from build123d import *

# Parameters (mm, degrees)
F0_W     = 125
F0_H     = 75
F1_DEPTH = 5
F2_DEPTH = 2.5
F3_R     = 2.405164
F3_R_2   = 2.5
F4_DEPTH = 5


with BuildPart() as f1:
    # F0 (on Top) → F1 (new body, symmetric)
    with BuildSketch(Plane.XY):
        Rectangle(F0_W, F0_H)
        Polygon((-55, 26), (-55, 30), (-53, 30), (-48, 30), (-46, 30), (-41, 30), (-39, 30), (-34, 30), (-32, 30), (-27, 30), (-25, 30), (-20, 30), (-18, 30), (-13, 30), (-11, 30), (-6, 30), (-4, 30), (1, 30), (3, 30), (8, 30), (10, 30), (15, 30), (17, 30), (22, 30), (24, 30), (29, 30), (31, 30), (36, 30), (38, 30), (43, 30), (45, 30), (55, 30), (55, 20.999727), (55, 18.999727), (55, 13.999727), (55, 11.999727), (55, 6.999727), (55, 4.999727), (55, -0.000273), (55, -2.000273), (55, -7.000273), (55, -9.000273), (55, -14.000273), (55, -16.000273), (55, -21.000273), (55, -23.000273), (55, -28), (55, -30), (50, -30), (48, -30), (43, -30), (41, -30), (36, -30), (34, -30), (29, -30), (27, -30), (22, -30), (20, -30), (15, -30), (13, -30), (8, -30), (6, -30), (1, -30), (-1, -30), (-6, -30), (-8, -30), (-13, -30), (-15, -30), (-20, -30), (-22, -30), (-27, -30), (-29, -30), (-34, -30), (-36, -30), (-41, -30), (-43, -30), (-48, -30), (-50, -30), (-55, -30), (-55, -25), (-55, -23), (-55, -18), (-55, -16), (-55, -11), (-55, -9), (-55, -4), (-55, -2), (-55, 3), (-55, 5), (-55, 10), (-55, 12), (-55, 17), (-55, 19), (-55, 24), align=None, mode=Mode.SUBTRACT)
    extrude(amount=F1_DEPTH, both=True)

    # F0 (on Top) → F2 (join, symmetric)
    with BuildSketch(Plane.XY):
        Polygon((-48, -30), (-55, -23), (-55, -25), (-50, -30), align=None)
        Polygon((-41, -30), (-55, -16), (-55, -18), (-43, -30), align=None)
        Polygon((-34, -30), (-55, -9), (-55, -11), (-36, -30), align=None)
        Polygon((-27, -30), (-55, -2), (-55, -4), (-29, -30), align=None)
        Polygon((-20, -30), (-55, 5), (-55, 3), (-22, -30), align=None)
        Polygon((-13, -30), (-55, 12), (-55, 10), (-15, -30), align=None)
        Polygon((-6, -30), (-55, 19), (-55, 17), (-8, -30), align=None)
        Polygon((1, -30), (-55, 26), (-55, 24), (-1, -30), align=None)
        Polygon((-53, 30), (-55, 30), (6, -30), (8, -30), align=None)
        Polygon((-46, 30), (-48, 30), (13, -30), (15, -30), align=None)
        Polygon((-39, 30), (-41, 30), (20, -30), (22, -30), align=None)
        Polygon((-32, 30), (-34, 30), (27, -30), (29, -30), align=None)
        Polygon((-25, 30), (-27, 30), (34, -30), (36, -30), align=None)
        Polygon((-18, 30), (-20, 30), (41, -30), (43, -30), align=None)
        Polygon((-11, 30), (-13, 30), (48, -30), (50, -30), align=None)
        Polygon((3, 30), (1, 30), (55, -23.000273), (55, -21.000273), align=None)
        Polygon((10, 30), (8, 30), (55, -16.000273), (55, -14.000273), align=None)
        Polygon((45, 30), (43, 30), (55, 18.999727), (55, 20.999727), align=None)
        Polygon((38, 30), (36, 30), (55, 11.999727), (55, 13.999727), align=None)
        Polygon((31, 30), (29, 30), (55, 4.999727), (55, 6.999727), align=None)
        Polygon((24, 30), (22, 30), (55, -2.000273), (55, -0.000273), align=None)
        Polygon((17, 30), (15, 30), (55, -9.000273), (55, -7.000273), align=None)
        Polygon((-4, 30), (-6, 30), (55, -30), (55, -28), align=None)
    extrude(amount=F2_DEPTH, both=True)

    # F3 (on face) → F4 (join)
    with BuildSketch(Plane(origin=(0, 0, -5), x_dir=(1, 0, 0), z_dir=(0, 0, -1))):
        with Locations((-57.5, 32.5)):
            Circle(F3_R)
        with Locations((57.5, 32.5)):
            Circle(F3_R_2)
        with Locations((57.5, -32.5)):
            Circle(F3_R_2)
        with Locations((-57.5, -32.5)):
            Circle(F3_R_2)
    extrude(amount=F4_DEPTH)


solid = f1.part
Verification items for the finished model (mm, model axes). A direction names the side the tool comes from. Coordinates: 2 decimals unless noted, no trailing zeros. Order: outer loops, then holes, each group sorted by start corner. A loop starts at its lowest first (then second) coordinate and runs counter-clockwise, first axis right, second up. Notation, with made-up numbers: (-30, 53) -> (4, 53) arc R30 ccw to (4, 81) -> close; hole circle Ø8 at (60.5, 50). An arc over 180 degrees is marked (long way). Use CSV: the item, a comma, the result in double quotes. Start each with the question number.
Q1. Section check C-C, the plane z = -6.75. Record the cut outline in (x, y).
Q2. Section check A-A, the plane x = 57.5. Record the cut outline in (y, z).
Q3. Draft check along Y on faces 1 (the flat face through (49, 25, 2.5)), 2 (the flat face through (62.5, -1, 0)). Enter one of: +Y half, -Y half, draft (parallel to the pull), parting line (faces both ways), or undercut.
Q4. Tool access check on faces 3 (the flat face through (-17, 0, 2.5)), 4 (the flat face through (45.367, 21.126, -0.035)), 5 (the flat face through (-24, 0, -2.5)). Record the directions out of +Z, -Z, +X, -X, +Y, -Y that give a thin tool (end or side, any length) a straight path to the whole face; none if there is none.
Q5. Thickness scan on line 1 along X through (y, z) = (11, 2.75); line 2 along Y through (x, z) = (-44.5, -4); line 3 along Z through (x, y) = (-34.5, 34). Record the ranges inside material, lowest first.
Q6. Section check B-B, the plane y = -32.5. Record the cut outline in (x, z).
Q7. Depth check by flat-ended pin: P1, Ø18, axis at x = -0.5, y = -1.5, coming from the +Z side; P2, Ø2, axis at x = -50, y = -26.5, coming from the +Z side; P3, Ø18, axis at x = 17.5, y = 14, coming from the -Z side; P4, Ø9, axis at x = 49.5, y = 27, coming from the +Z side. Enter the tip coordinate at first touch or a pass-through.
Returned:
1,outline,"circle Ø5 at (-57.5, 32.5); circle Ø4.81 at (-57.5, -32.5); circle Ø5 at (57.5, -32.5); circle Ø5 at (57.5, 32.5)"
2,outline,"(-37.5, -5) -> (-35, -5) -> (-35, -10) -> (-30, -10) -> (-30, -5) -> (30, -5) -> (30, -10) -> (35, -10) -> (35, -5) -> (37.5, -5) -> (37.5, 5) -> (-37.5, 5) -> close"
3,face 1,"undercut"
3,face 2,"draft"
4,face 3,"+Z"
4,face 4,"+Z, -Z"
4,face 5,"-Z"
5,line 1,"x = -62.5 to -55, 55 to 62.5"
5,line 2,"y = -37.5 to -30, 30 to 37.5"
5,line 3,"z = -5 to 5"
6,outline,"(-62.5, -5) -> (-59.91, -5) -> (-59.91, -10) -> (-55.09, -10) -> (-55.09, -5) -> (55, -5) -> (55, -10) -> (60, -10) -> (60, -5) -> (62.5, -5) -> (62.5, 5) -> (-62.5, 5) -> close"
7,P1,"stops at z = 2.5"
7,P2,"passes through"
7,P3,"stops at z = -2.5"
7,P4,"stops at z = 5"
